Verification items for the finished model (mm, model axes). Face numbers are marked on the shaded views. A direction names the side the tool comes from. Give positions to 0.01 mm unless a question says otherwise; leave off trailing zeros. Write each loop counter-clockwise with the first axis right and the second up, starting at its lowest first coordinate (ties: lowest second). Pieces come first, ordered by that corner, then holes. Notation, with made-up numbers: (60, 52.5) -> (117, 52.5) arc R18 ccw to (117, 79.5) -> close; hole circle Ø2 at (89, 48.5). An arc over 180 degrees is marked (long way). Use one line per item in the form item = value. Start each with the question number.
(1) Section check D-D, the plane y = 5. State how many separate pieces and enclosed holes the cut face has, plus the area to 3 significant figures.
(2) Depth check by flat-ended pin: pin 1 Ø2 at (x, y) = (11.5, 2.5) entering from +Z; pin 2 Ø1.5 at (x, z) = (35, -19) entering from +Y; pin 3 Ø3 at (x, z) = (-37.5, 15.5) entering from +Y; pin 4 Ø5 at (y, z) = (9, -12) entering from +X. Enter the tip coordinate at first touch or a pass-through.
(3) Section check A-A, the plane z = 15.5. Record the cut outline in (x, y), plus the area to 3 significant figures.
(4) Section check B-B, the plane z = 9. Record the cut outline in (x, y), plus the area to 3 significant figures.
(5) Section check C-C, the plane y = 18.5. Record the cut outline in (x, z), plus the area to 3 significant figures.
(6) Set-up check for the marked faces 1 and 2: record each of +Z, -Z, +X, -X, +Y, -Y from which the full face is reachable in a straight line by a thin tool's end or side.
(7) Release check for a two-part mould opening along Z. For the marked faces 3, 4 and 5 record: pulls with the +Z half, pulls with the -Z half, needs draft (parallel to the pull), parting line crosses it, or undercut.
(8) Scan lines: L1, parallel to X at y = 4, z = -15; L2, parallel to X at y = 6.25, z = 15.5; L3, parallel to Z at x = 21.5, y = 7. Record each from-to range of solid material in increasing order.
from build123d import *

# Parameters (mm, degrees)
SKETCH1_W               = 100
SKETCH1_H               = 65.435021842
SKETCH1_R               = 1.2499975
SKETCH1_W_2             = 71.5
SKETCH1_H_2             = 26.5
BOSS_EXTRUDE1_DEPTH     = 7.5
MIRROR2_OUTLINE_R       = 1.2499975
MIRROR2_DEPTH           = 7.5
MIRROR3_OUTLINE_R       = 1.2499975
MIRROR3_DEPTH           = 7.5
BOSS_EXTRUDE2_DEPTH     = 100
FILLET2_R               = 7.5
CUT_EXTRUDE2_DEPTH      = 116.441064867
CUT_EXTRUDE2_DEPTH_BACK = 116.441064867
SKETCH5_W               = 7.5
SKETCH5_H               = 10.864122905
BOSS_EXTRUDE3_DEPTH     = 100
FILLET4_R               = 3.5
FILLET5_R               = 7.5
FILLET6_R               = 5


# Read off the part's stored shape, not the designer's step: Mirror2, Mirror3
with BuildPart() as part:
    # Sketch1 → Boss-Extrude1 (new body)
    with BuildSketch(Plane(origin=(0, 0, 0), x_dir=(1, 0, 0), z_dir=(0, 1, 0))):
        Rectangle(SKETCH1_W, SKETCH1_H)
        with Locations(Location((-37.5, 15.499999988, 0), (0, 0, 270))):
            Circle(SKETCH1_R, mode=Mode.SUBTRACT)
        Rectangle(SKETCH1_W_2, SKETCH1_H_2, mode=Mode.SUBTRACT)
    extrude(amount=BOSS_EXTRUDE1_DEPTH)

    # Mirror2 outline → Mirror2 (cut)
    with BuildSketch(Plane(origin=(0, 0, 0), x_dir=(1, 0, 0), z_dir=(0, 1, 0))):
        with Locations((37.5, 15.499999988)):
            Circle(MIRROR2_OUTLINE_R)
    extrude(amount=MIRROR2_DEPTH, mode=Mode.SUBTRACT)

    # Mirror3 outline → Mirror3 (cut)
    with BuildSketch(Plane(origin=(0, 0, 0), x_dir=(1, 0, 0), z_dir=(0, 1, 0))):
        with Locations((-37.5, -15.499999988)):
            Circle(MIRROR3_OUTLINE_R)
        with Locations((37.5, -15.499999988)):
            Circle(MIRROR3_OUTLINE_R)
    extrude(amount=MIRROR3_DEPTH, mode=Mode.SUBTRACT)

    # Sketch4 → Boss-Extrude2 (add)
    with BuildSketch(Plane(origin=(50, 0, 0), x_dir=(0, 0, -1), z_dir=(1, 0, 0))):
        Polygon((28.324112639, 0), (8.64916927, 47.499515121), (16.14916927, 47.499515121), (32.717510921, 7.5), (35.824112639, 0), align=None)
    extrude(amount=-BOSS_EXTRUDE2_DEPTH)

    # Fillet2
    fillet2_edges = [part.edges().sort_by_distance(p)[0] for p in [
        (0, 0, -35.824112639),
    ]]
    fillet(fillet2_edges, radius=FILLET2_R)

    # Sketch5 → Cut-Extrude2 (cut, two sides: drawn at the far end of the back side and taken through both)
    with BuildSketch(Plane(origin=(50, 0, 0), x_dir=(0, 0, -1), z_dir=(1, 0, 0)).offset(-CUT_EXTRUDE2_DEPTH_BACK)):
        with Locations((-30.896013204, 2.067938548)):
            Rectangle(SKETCH5_W, SKETCH5_H)
    extrude(amount=CUT_EXTRUDE2_DEPTH + CUT_EXTRUDE2_DEPTH_BACK, mode=Mode.SUBTRACT)

    # Sketch6 → Boss-Extrude3 (add)
    with BuildSketch(Plane(origin=(50, 0, 0), x_dir=(0, 0, -1), z_dir=(1, 0, 0))):
        Polygon((-27.146013204, 0), (-32.146013204, 0), (-32.146013204, 38.274911515), (12.337893428, 56.700748949), (13.485305965, 53.930650039), (16.14916927, 47.499515121), (12.93914216, 38.274911515), (8.66493866, 47.461444446), (7.84966016, 49.429700857), (-27.146013204, 34.934018325), align=None)
    extrude(amount=-BOSS_EXTRUDE3_DEPTH)

    # Fillet4
    fillet4_edges = [part.edges().sort_by_distance(p)[0] for p in [
        (0, 7.5, -25.217510921),
    ]]
    fillet(fillet4_edges, radius=FILLET4_R)

    # Fillet5
    fillet5_edges = [part.edges().sort_by_distance(p)[0] for p in [
        (0, 7.5, 27.146013204),
        (0, 0, 32.146013204),
    ]]
    fillet(fillet5_edges, radius=FILLET5_R)

    # Fillet6
    fillet6_edges = [part.edges().sort_by_distance(p)[0] for p in [
        (0, 34.934018325, 27.146013204),
        (0, 38.274911515, 32.146013204),
        (0, 56.700748949, -12.337893428),
        (0, 49.429700857, -7.84966016),
    ]]
    fillet(fillet6_edges, radius=FILLET6_R)


solid = part.part
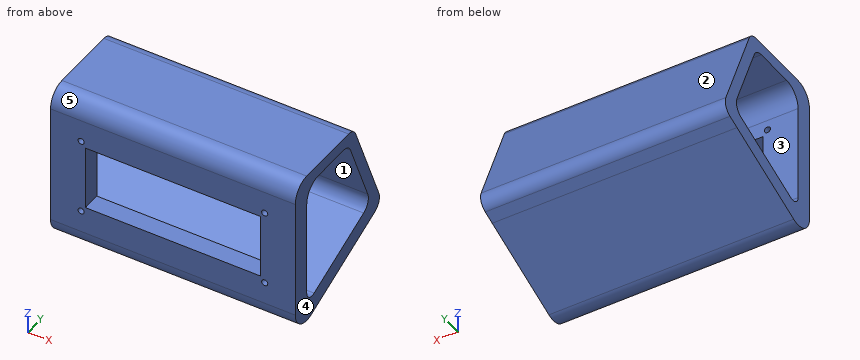
Completed:
q1.separate_pieces = 1
q1.enclosed_holes = 5
q1.area = 4,420 mm²
q2.pin_1 = 30.99
q2.pin_2 = 42.43
q2.pin_3 = 45.79
q2.pin_4 = 50
q3.outline = (-50, 0) -> (-38.75, 0) -> (-38.75, 7.5) -> (-50, 7.5) -> close; (-50, 39.76) -> (50, 39.76) -> (50, 45.17) -> (-50, 45.17) -> close; (-36.25, 0) -> (36.25, 0) -> (36.25, 7.5) -> (-36.25, 7.5) -> close; (38.75, 0) -> (50, 0) -> (50, 7.5) -> (38.75, 7.5) -> close
q3.area = 1,250 mm²
q4.outline = (-50, 0) -> (-35.75, 0) -> (-35.75, 7.5) -> (-50, 7.5) -> close; (-50, 42.45) -> (50, 42.45) -> (50, 47.86) -> (-50, 47.86) -> close; (35.75, 0) -> (50, 0) -> (50, 7.5) -> (35.75, 7.5) -> close
q4.area = 755 mm²
q5.outline = (-50, -28.16) -> (50, -28.16) -> (50, -20.66) -> (-50, -20.66) -> close; (-50, 27.15) -> (50, 27.15) -> (50, 32.15) -> (-50, 32.15) -> close
q5.area = 1,250 mm²
q6.face_1 = +X, -X
q6.face_2 = +Z, +X, -X, +Y
q7.face_3 = undercut
q7.face_4 = needs draft
q7.face_5 = pulls with the +Z half
q8.L1 = -50 to -38.65, -36.35 to 36.35, 38.65 to 50
q8.L2 = -50 to -38.75, -36.25 to 36.25, 38.75 to 50
q8.L3 = -32.08 to -13.25, 13.25 to 32.13
